Design review of the part shown in the three views and the two pictorial views. Dimensions are in mm from the part's minimum x, y and z. Give positions to 0.01 mm unless a question says otherwise; leave off trailing zeros. Order: outer loops, then holes, each group sorted by start corner. A loop starts at its lowest first (then second) coordinate and runs counter-clockwise, first axis right, second up.
Item 1: Consider section B-B (z = 1.45). Give the boundary of the cut face in (x, y), plus the area to 3 significant figures.
Item 2: For P1, Ø5, axis at x = 31, y = 8.5, coming from the -Z side; P2, Ø1, axis at x = 10.5, z = 0.5, coming from the +Y side; P3, Ø3, axis at y = 3.5, z = 0.5, coming from the -X side, all flat-tipped, find the tip position at first contact; note any pin that passes through.
Item 3: For probe 1 along X at (y, z) = (6.25, 2.15); probe 2 along Y at (x, z) = (28.5, 3.9) (1 decimal); probe 3 along X at (y, z) = (2, 0.55), list the stretches that pass through material, from the lowest coordinate up.
Item 4: Consider section A-A (y = 9.25). Give the boundary of the cut face in (x, z), plus the area to 3 significant figures.
Item 5: Consider section D-D (y = 7.25). Give the boundary of the cut face in (x, z).
Item 6: Consider section C-C (x = 8.5). Give the boundary of the cut face in (y, z), plus the area to 3 significant figures.
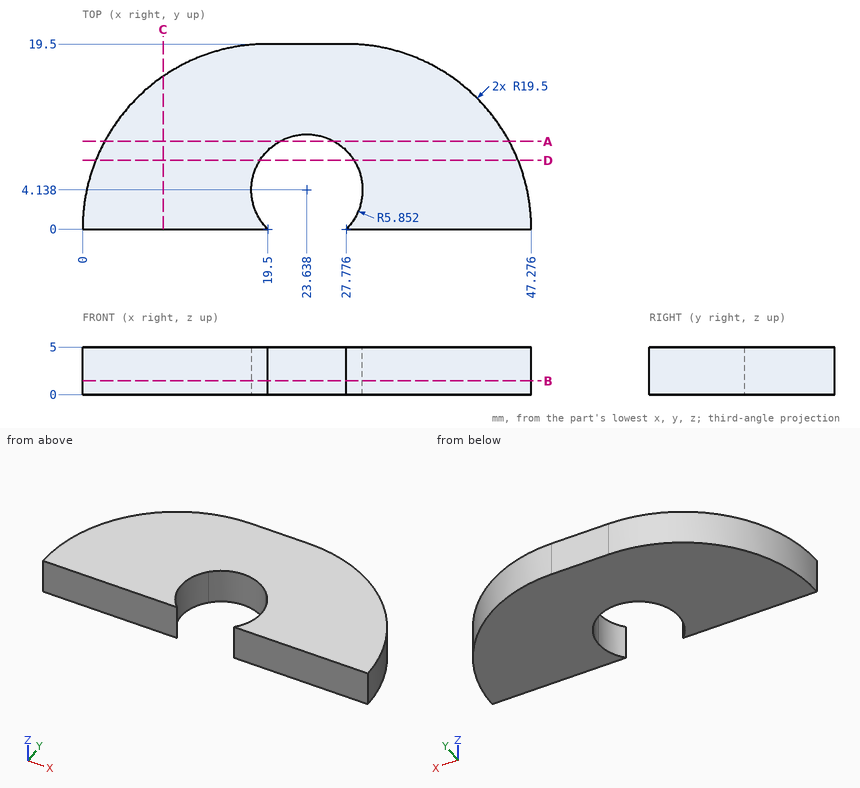
Resolved:
1. outline: (0, 0) - (19.5, 0) arc R5.85 cw (long way) to (27.78, 0) - (47.28, 0) arc R19.5 ccw to (27.78, 19.5) - (19.5, 19.5) arc R19.5 ccw to start
1. area: 661 mm2
2. P1: stops at z = 0
2. P2: stops at y = 17.55
2. P3: stops at x = 0.1
3. probe 1: x = 1.03 to 18.18, 29.1 to 46.25
3. probe 2: y = 0 to 0.9, 7.4 to 19.5
3. probe 3: x = 0.1 to 18.19, 29.09 to 47.17
4. outline: (2.33, 0) - (20.79, 0) - (20.79, 5) - (2.33, 5) - close; (26.49, 0) - (44.94, 0) - (44.94, 5) - (26.49, 5) - close
4. area: 185 mm2
5. outline: (1.4, 0) - (18.68, 0) - (18.68, 5) - (1.4, 5) - close; (28.59, 0) - (45.88, 0) - (45.88, 5) - (28.59, 5) - close
6. outline: (0, 0) - (16.1, 0) - (16.1, 5) - (0, 5) - close
6. area: 80.5 mm2
